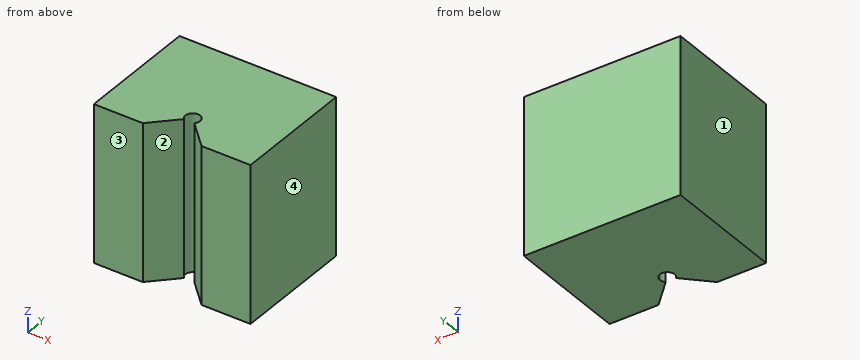
from build123d import *

# Parameters (mm, degrees)
F0_W     = 32
F0_H     = 32
F1_DEPTH = 25
F3_DEPTH = 32.001


with BuildPart() as f1:
    # F0 (on Front) → F1 (new body)
    with BuildSketch(Plane.XZ):
        Rectangle(F0_W, F0_H)
    extrude(amount=-F1_DEPTH)

    # F2 (on face) → F3 (cut, through all)
    with BuildSketch(Plane.XY.offset(16)):
        with BuildLine():
            Line((-1.0606601718, 4.9393398282), (-6, 0))
            Line((-6, 0), (6, 0))
            Line((6, 0), (1.0606601718, 4.9393398282))
            ThreePointArc((1.0606601718, 4.9393398282), (0, 4.5), (-1.0606601718, 4.9393398282))
        make_face()
        with BuildLine():
            ThreePointArc((1.5, 6), (-0.5740251485, 7.3858192988), (-1.0606601718, 4.9393398282))
            Line((-1.0606601718, 4.9393398282), (0, 6))
            Line((0, 6), (1.0606601718, 4.9393398282))
            ThreePointArc((1.0606601718, 4.9393398282), (1.3858192988, 5.4259748515), (1.5, 6))
        make_face()
        with BuildLine():
            Line((0, 6), (-1.0606601718, 4.9393398282))
            ThreePointArc((-1.0606601718, 4.9393398282), (0, 4.5), (1.0606601718, 4.9393398282))
            Line((1.0606601718, 4.9393398282), (0, 6))
        make_face()
    extrude(amount=-F3_DEPTH, mode=Mode.SUBTRACT)


solid = f1.part
Check sheet for the modelled part. Datum: model origin and axes. Units: mm. Face numbers are marked on the shaded views. Give positions to 0.01 mm unless a question says otherwise; leave off trailing zeros. Write each loop counter-clockwise with the first axis right and the second up, starting at its lowest first coordinate (ties: lowest second). Pieces come first, ordered by that corner, then holes. Notation, with made-up numbers: M 38.5,6.5 L 47.5,6.5 A24 ccw 47.5,40.5 Z; hole C 47,78 d3. An arc over 180 degrees is marked long. Use one line per item in the form item = value.
(1) Depth check by flat-ended pin: P1, Ø8, axis at x = -8, z = -11.5, coming from the -Y side. Enter the tip coordinate at first touch or a pass-through.
Answer block:
P1 = 0
(2) Material ranges on line 1 along X through (y, z) = (6, -5.5); line 2 along Y through (x, z) = (0, 2); line 3 along Y through (x, z) = (-3, -2.5), recorded low to high.
Answer block:
line_1 = -16 to -1.5, 1.5 to 16
line_2 = 7.5 to 25
line_3 = 3 to 25
(3) Section check C-C on x = 0. Record the boundary of the cut face in (y, z), plus the area to 3 significant figures.
Answer block:
outline = M 7.5,-16 L 25,-16 L 25,16 L 7.5,16 Z
area = 560 mm2
(4) Draft check along X on the marked faces 1, 2, 3 and 4. Enter one of: pulls with the +X half, pulls with the -X half, needs draft (parallel to the pull), parting line crosses it, or undercut.
Answer block:
face_1 = pulls with the -X half
face_2 = undercut
face_3 = needs draft
face_4 = pulls with the +X half
(5) Section check B-B on z = 7. Record the boundary of the cut face in (x, y), plus the area to 3 significant figures.
Answer block:
outline = M -16,0 L -6,0 L -1.06,4.94 A1.5 cw long 1.06,4.94 L 6,0 L 16,0 L 16,25 L -16,25 Z
area = 759 mm2
(6) Section check A-A on y = 3. Record the boundary of the cut face in (x, z), plus the area to 3 significant figures.
Answer block:
outline = M -16,-16 L -3,-16 L -3,16 L -16,16 Z; M 3,-16 L 16,-16 L 16,16 L 3,16 Z
area = 832 mm2
